Geometry: final body of the model. Coordinates: model frame, mm. A direction names the side the tool comes from. Give positions to 0.01 mm unless a question says otherwise; leave off trailing zeros. Write each loop counter-clockwise with the first axis right and the second up, starting at its lowest first coordinate (ties: lowest second). Pieces come first, ordered by that corner, then holes.
```python
from build123d import *

# Parameters (mm, degrees)
BOSS_EXTRUDE2_DEPTH = 6.35
SKETCH4_R           = 2.3
SKETCH4_R_2         = 3.81
CUT_EXTRUDE1_DEPTH  = 12.7
CUT_EXTRUDE2_DEPTH  = 3.81


with BuildPart() as part:
    # Sketch3 → Boss-Extrude2 (new body)
    with BuildSketch(Plane(origin=(0, 0, 0), x_dir=(1, 0, 0), z_dir=(0, 1, 0))):
        with BuildLine():
            Line((-9.525, 11.25), (9.525, 11.25))
            ThreePointArc((9.525, 11.25), (14.740696218, 0), (9.525, -11.25))
            Line((9.525, -11.25), (-9.525, -11.25))
            ThreePointArc((-9.525, -11.25), (-14.740696218, 0), (-9.525, 11.25))
        make_face()
    extrude(amount=BOSS_EXTRUDE2_DEPTH)

    # Sketch4 → Cut-Extrude1 (cut)
    with BuildSketch(Plane(origin=(0, 6.35, 0), x_dir=(1, 0, 0), z_dir=(0, 1, 0))):
        with Locations((-8.89, 3.81)):
            Circle(SKETCH4_R)
        with Locations((-8.89, -3.81)):
            Circle(SKETCH4_R)
        with Locations((9.525, 0)):
            Circle(SKETCH4_R_2)
    extrude(amount=-CUT_EXTRUDE1_DEPTH, mode=Mode.SUBTRACT)

    # Sketch5 → Cut-Extrude2 (cut)
    with BuildSketch(Plane.XZ):
        with BuildLine():
            Line((9.525, 11.25), (3.175, 11.25))
            Line((3.175, 11.25), (3.175, -11.25))
            Line((3.175, -11.25), (9.525, -11.25))
            ThreePointArc((9.525, -11.25), (14.740696218, 0), (9.525, 11.25))
        make_face()
    extrude(amount=-CUT_EXTRUDE2_DEPTH, mode=Mode.SUBTRACT)


solid = part.part
```
Item 1: Section C-C, the plane y = 4.25. Return the cut outline in (x, z) (3 decimals), plus the area to 3 significant figures.
Found:
outline: (-9.525, -11.25) - (9.525, -11.25) arc R14.741 ccw to (9.525, 11.25) - (-9.525, 11.25) arc R14.741 ccw to start; hole circle Ø4.6 at (-8.89, -3.81); hole circle Ø4.6 at (-8.89, 3.81); hole circle Ø7.62 at (9.525, 0)
area: 513 mm2
Item 2: Pull-direction query (X, two-part tool) for faces 1 (the face through (5.72, 5.1, -0.17)), 2 (the face through (-14.74, 3.13, 0.18)), 3 (the face through (-4, 0, 0)); classes: +X half, -X half, draft (parallel to the pull), parting line (faces both ways), or undercut.
Found:
face 1: undercut
face 2: -X half
face 3: draft
Item 3: Section A-A, the plane z = 0. Return the cut outline in (x, y) (3 decimals), plus the area to 3 significant figures.
Found:
outline: (-14.741, 0) - (3.175, 0) - (3.175, 3.81) - (5.715, 3.81) - (5.715, 6.35) - (-14.741, 6.35) - close; (13.335, 3.81) - (14.741, 3.81) - (14.741, 6.35) - (13.335, 6.35) - close
area: 124 mm2
Item 4: Section D-D, the plane y = 0.75. Return the cut outline in (x, z) (3 decimals).
Found:
outline: (-9.525, -11.25) - (3.175, -11.25) - (3.175, 11.25) - (-9.525, 11.25) arc R14.741 ccw to start; hole circle Ø4.6 at (-8.89, -3.81); hole circle Ø4.6 at (-8.89, 3.81)
Item 5: Pin query (flat end, axial travel): pin 1 Ø3 at (x, z) = (-8.89, -3.81) entering from -Y; pin 2 Ø1.5 at (x, y) = (-11, 4) entering from -Z; pin 3 Ø1.1 at (y, z) = (2.5, -0.5) entering from +X (3 decimals); pin 4 Ø9.5 at (x, z) = (10.5, 4) entering from -Y. Return the tip coordinate at first contact, or that it passes through.
Found:
pin 1: passes through
pin 2: stops at z = -10.59
pin 3: stops at x = 3.175
pin 4: stops at y = 3.81
Item 6: Line query: L1, parallel to Z at x = -8.89, y = 2.75; L2, parallel to X at y = 5.75, z = -3.25; L3, parallel to Z at x = -9.5, y = 2.5. Output: solid intervals per line, ascending.
Found:
L1: z = -11.25 to -6.11, -1.51 to 1.51, 6.11 to 11.25
L2: x = -14.38 to -11.12, -6.66 to 7.54, 11.51 to 14.38
L3: z = -11.25 to -6.03, -1.59 to 1.59, 6.03 to 11.25
Item 7: Reachability of faces 4 (the face through (14.74, 5.06, -0.18)), 5 (the face through (3.175, 2, 0)) from +Z, -Z, +X, -X, +Y, -Y: full face, straight path, thin tool, end or side. Return the list, or none.
Found:
face 4: +X, +Y, -Y
face 5: +Z, -Z, +X, -Y
Item 8: Section B-B, the plane x = -8.89. Return the cut outline in (y, z), plus the area to 3 significant figures.
Found:
outline: (0, -11.25) - (6.35, -11.25) - (6.35, -6.11) - (0, -6.11) - close; (0, -1.51) - (6.35, -1.51) - (6.35, 1.51) - (0, 1.51) - close; (0, 6.11) - (6.35, 6.11) - (6.35, 11.25) - (0, 11.25) - close
area: 84.5 mm2
